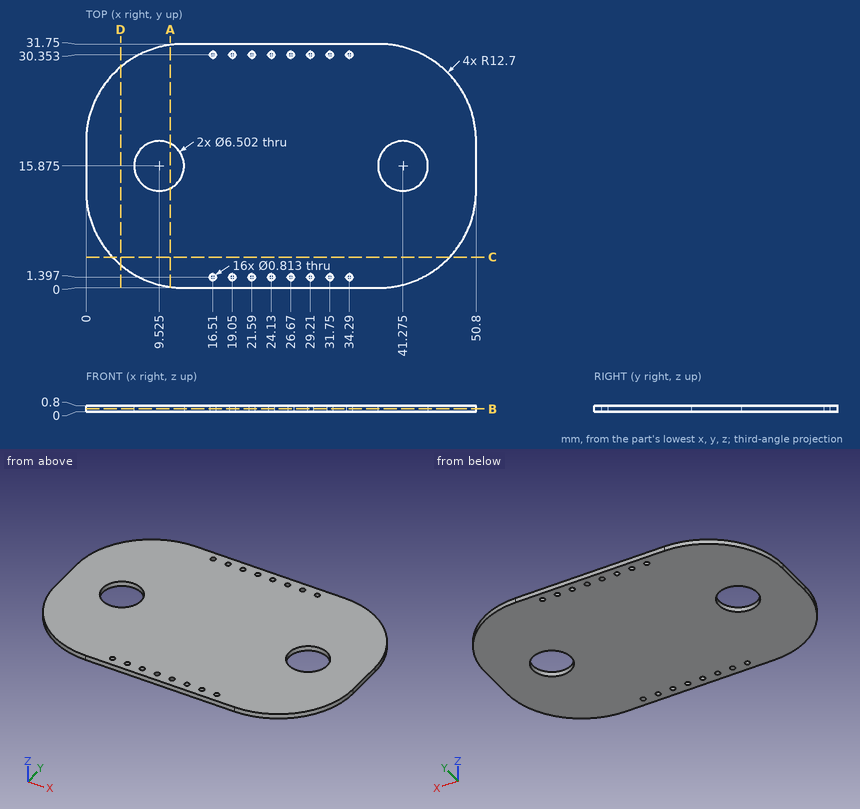
Part print with two shaded views. Sizes in mm from the minimum x, y, z corner. Coordinates: 2 decimals unless noted, no trailing zeros. Write each loop counter-clockwise with the first axis right and the second up, starting at its lowest first coordinate (ties: lowest second). Pieces come first, ordered by that corner, then holes. Notation, with made-up numbers: (2, 88.25) - (54, 88.25) arc R19 cw to (54, 94.25) - close; hole circle Ø11 at (4.5, 53). An arc over 180 degrees is marked (long way). Put each result on its own line as item: value.
1. Band-saw the part on A-A (x = 11). Write the cut outline in (y, z) (1 decimal).
Final values:
outline: (0.1, 0) - (13, 0) - (13, 0.8) - (0.1, 0.8) - close; (18.8, 0) - (31.6, 0) - (31.6, 0.8) - (18.8, 0.8) - close
2. Flat gauge pin, fed straight in: pin 1 Ø4 at (x, y) = (9.525, 15.875) entering from +Z. Where does the tip first touch, or does it go through?
Final values:
pin 1: passes through
3. Probe line 1 along Y through (x, z) = (26.67, 0.3); line 2 along X through (y, z) = (18, 0.55) (1 decimal); line 3 along X through (y, z) = (15, 0.3) (1 decimal). List the from-to ranges inside material, lowest first. Write a range as [from, to].
Final values:
line 1: y = [0, 0.99], [1.8, 29.95], [30.76, 31.75]
line 2: x = [0, 7.1], [12, 38.8], [43.7, 50.8]
line 3: x = [0, 6.4], [12.7, 38.1], [44.4, 50.8]
4. Band-saw the part on B-B (z = 0.4). Give the number of separate pieces and of enclosed holes in the cut face, then the cut area to 3 significant figures.
Final values:
separate pieces: 1
enclosed holes: 18
area: 1,400 mm²
5. Band-saw the part on C-C (y = 4). Write the cut outline in (x, z).
Final values:
outline: (3.45, 0) - (47.35, 0) - (47.35, 0.8) - (3.45, 0.8) - close
6. Band-saw the part on D-D (x = 4.5). Write the cut outline in (y, z).
Final values:
outline: (3, 0) - (28.75, 0) - (28.75, 0.8) - (3, 0.8) - close
